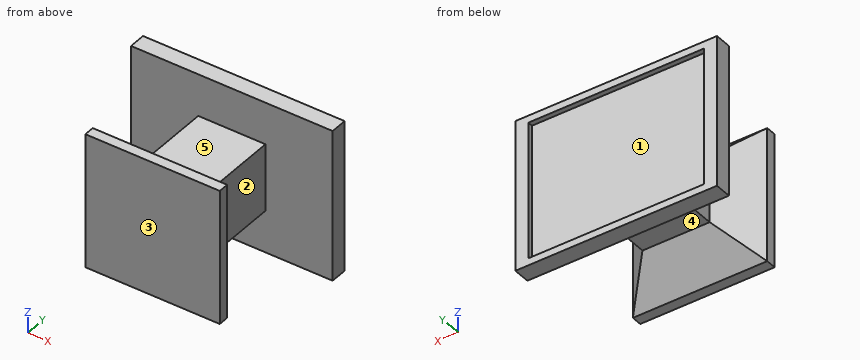
from build123d import *

# Parameters (mm, degrees)
SKETCH1_W           = 39
SKETCH1_H           = 29.25
BOSS_EXTRUDE1_DEPTH = 3.25
SKETCH3_W           = 13
SKETCH3_H           = 13
BOSS_EXTRUDE3_DEPTH = 13
SKETCH5_W           = 34
SKETCH5_H           = 24
CUT_EXTRUDE1_DEPTH  = 1
SKETCH6_W           = 26
SKETCH6_H           = 26
BOSS_EXTRUDE4_DEPTH = 2
SKETCH8_W           = 34
SKETCH8_H           = 1.25
CUT_EXTRUDE2_DEPTH  = 1


with BuildPart() as part:
    # Sketch1 → Boss-Extrude1 (new body)
    with BuildSketch(Plane(origin=(0, 0, 0), x_dir=(1, 0, 0), z_dir=(0, 1, 0))):
        Rectangle(SKETCH1_W, SKETCH1_H)
    extrude(amount=BOSS_EXTRUDE1_DEPTH)

    # Sketch3 → Boss-Extrude3 (add)
    with BuildSketch(Plane.XZ):
        Rectangle(SKETCH3_W, SKETCH3_H)
    extrude(amount=BOSS_EXTRUDE3_DEPTH)

    # Sketch4 → section 0 of loft1
    with BuildSketch(Plane(origin=(0, -19.5, 0), x_dir=(-1, 0, 0), z_dir=(0, -1, 0)), mode=Mode.PRIVATE) as loft1_s0:
        with BuildLine():
            Line((-13, 13), (13, 13))
            Line((13, 13), (13, -13))
            Line((13, -13), (-13, -13))
            Line((-13, -13), (-13, 13))
        make_face()
    # loft up to a face of the part (loft1)
    loft([loft1_s0.sketch, part.faces().sort_by_distance((0, -13, 0))[0]])

    # Sketch5 → Cut-Extrude1 (cut)
    with BuildSketch(Plane(origin=(0, 3.25, 0), x_dir=(1, 0, 0), z_dir=(0, 1, 0))):
        Rectangle(SKETCH5_W, SKETCH5_H)
    extrude(amount=-CUT_EXTRUDE1_DEPTH, mode=Mode.SUBTRACT)

    # Sketch6 → Boss-Extrude4 (add)
    with BuildSketch(Plane.XZ.offset(19.5)):
        Rectangle(SKETCH6_W, SKETCH6_H)
    extrude(amount=BOSS_EXTRUDE4_DEPTH)

    # Sketch8 → Cut-Extrude2 (cut)
    with BuildSketch(Plane(origin=(0, 3.25, 0), x_dir=(1, 0, 0), z_dir=(0, 1, 0))):
        with Locations((0, -12.625)):
            Rectangle(SKETCH8_W, SKETCH8_H)
    cut_extrude2 = extrude(amount=-CUT_EXTRUDE2_DEPTH, mode=Mode.SUBTRACT)

    # Mirror1: Cut-Extrude2 across plane
    add(cut_extrude2.mirror(Plane.XY), mode=Mode.SUBTRACT)


solid = part.part
Source: CAD feature listing. Evaluate the final solid. Frame: model axes, mm. Face numbers are marked on the shaded views. A direction names the side the tool comes from. Give positions to 0.01 mm unless a question says otherwise; leave off trailing zeros. Loops run counter-clockwise (first coordinate to the right, second up) from the corner with the lowest first, then second, coordinate; pieces in that order, holes last. Notation, with made-up numbers: (65, 46.5) -> (83, 46.5) arc R26 ccw to (83, 79.5) -> close; hole circle Ø9 at (20, 78). An arc over 180 degrees is marked (long way). Use a Markdown table: item, result. Add a question column.
1) First-contact query: pin 1 (4 mm diameter, centred on x = 3, y = -4.5, fed in from +Z); pin 2 (1.6 mm diameter, centred on x = 3, y = -20.5, fed in from -Z); pin 3 (3 mm diameter, centred on y = -14, z = 0.5, fed in from -X). Flat tips, straight axial feed; report the tip coordinate or a pass-through.
2) Reachability of the marked faces 4 and 5 from +Z, -Z, +X, -X, +Y, -Y: full face, straight path, thin tool, end or side. Return the list, or none.
3) Section query A-A, the plane y = -6.5. Return the cut outline in (x, z).
4) Line query: line 1 along Y through (x, z) = (2.5, -2.25); line 2 along Y through (x, z) = (1, -11.5); line 3 along Y through (x, z) = (-11, -11). Output: solid intervals per line, ascending. Write a range as [from, to].
5) Pull-direction query (X, two-part tool) for the marked faces 1, 2 and 3; classes: +X half, -X half, draft (parallel to the pull), parting line (faces both ways), or undercut.
Numbers:
| question | item | result |
|---|---|---|
| 1 | pin 1 | stops at z = 6.5 |
| 1 | pin 2 | stops at z = -13 |
| 1 | pin 3 | stops at x = -9 |
| 2 | face 4 | -Z, +X, -X |
| 2 | face 5 | +Z, +X, -X |
| 3 | outline | (-6.5, -6.5) -> (6.5, -6.5) -> (6.5, 6.5) -> (-6.5, 6.5) -> close |
| 4 | line 1 | y = [-21.5, 2.25] |
| 4 | line 2 | y = [-21.5, -18], [0, 2.25] |
| 4 | line 3 | y = [-21.5, -17.5], [0, 2.25] |
| 5 | face 1 | undercut |
| 5 | face 2 | +X half |
| 5 | face 3 | draft |
